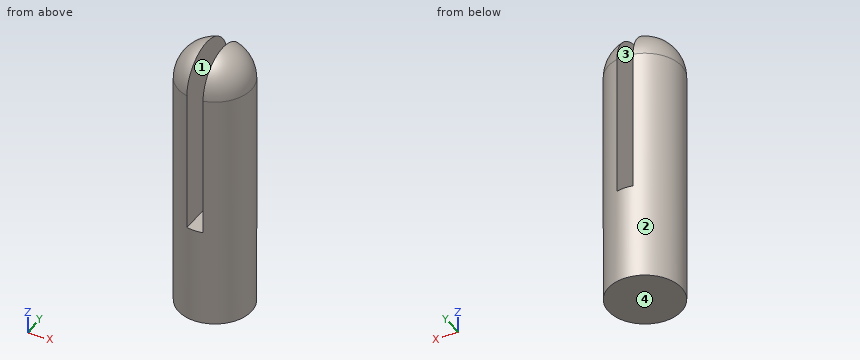
from build123d import *

# Parameters (mm, degrees)
SKETCH1_R           = 45
BOSS_EXTRUDE1_DEPTH = 340
FILLET1_R           = 45
SKETCH2_OUTSIDE_W   = 414.608
SKETCH2_OUTSIDE_H   = 164.608
SKETCH2_OUTSIDE_W_2 = 150
SKETCH2_OUTSIDE_H_2 = 90
CUT_EXTRUDE1_DEPTH  = 10


with BuildPart() as part:
    # Sketch1 → Boss-Extrude1 (new body)
    with BuildSketch(Plane.XY):
        Circle(SKETCH1_R)
    extrude(amount=BOSS_EXTRUDE1_DEPTH)

    # Fillet1
    fillet1_edges = [part.edges().sort_by_distance(p)[0] for p in [
        (-45, 0, 340),
    ]]
    fillet(fillet1_edges, radius=FILLET1_R)

    # Sketch2 outside → Cut-Extrude1 (cut, symmetric)
    with BuildSketch(Plane(origin=(0, 0, 0), x_dir=(0, 0, -1), z_dir=(1, 0, 0))):
        with Locations((-170, 0)):
            Rectangle(SKETCH2_OUTSIDE_W, SKETCH2_OUTSIDE_H)
        with Locations((-45, 0)):
            Rectangle(SKETCH2_OUTSIDE_W_2, SKETCH2_OUTSIDE_H_2, mode=Mode.SUBTRACT)
    extrude(amount=CUT_EXTRUDE1_DEPTH, both=True, mode=Mode.SUBTRACT)


solid = part.part
For this review, take the finished solid that the model builds, in its own axes (mm). Face numbers are marked on the shaded views. Coordinates: 2 decimals unless noted, no trailing zeros. Order: outer loops, then holes, each group sorted by start corner. A loop starts at its lowest first (then second) coordinate and runs counter-clockwise, first axis right, second up. Notation, with made-up numbers: (-15, 59.5) - (29, 59.5) arc R26 cw to (29, 77.5) - close; hole circle Ø9 at (54, 53.25). An arc over 180 degrees is marked (long way). Use one line per item in the form item = value.
Q1. Draft analysis for pull direction X (two halves, no side actions). For the marked faces 1, 2, 3 and 4, state which applies: +X half, -X half, draft (parallel to the pull), parting line (faces both ways), or undercut.
Checked values:
face_1 = undercut
face_2 = parting line
face_3 = undercut
face_4 = draft
Q2. Consider section A-A (y = 0). Give the boundary of the cut face in (x, z).
Checked values:
outline = (-45, 0) - (45, 0) - (45, 295) arc R45 ccw to (10, 338.87) - (10, 120) - (-10, 120) - (-10, 338.87) arc R45 ccw to (-45, 295) - close
Q3. For P1, Ø4, axis at x = -14.5, y = 21, coming from the -Z side; P2, Ø1.5, axis at x = -4, y = -25, coming from the +Z side; P3, Ø6, axis at x = 10, z = 34.5, coming from the +Y side; P4, Ø3, axis at x = -15.5, y = -29, coming from the +Z side, all flat-tipped, find the tip position at first contact; note any pin that passes through.
Checked values:
P1 = 0
P2 = 120
P3 = 44.45
P4 = 327.25
Q4. Consider section B-B (z = 209). Give the boundary of the cut face in (x, y).
Checked values:
outline = (-10, -43.87) - (-10, 43.87) arc R45 ccw to start; (10, -43.87) arc R45 ccw to (10, 43.87) - close
Q5. For probe 1 along X at (y, z) = (1, 166.5); probe 2 along X at (y, z) = (32, 149.5); probe 3 along Z at (x, y) = (1, 1), list the stretches that pass through material, from the lowest coordinate up. Write a range as from..to.
Checked values:
probe_1 = -44.99..-10, 10..44.99
probe_2 = -31.64..-10, 10..31.64
probe_3 = 0..120
Q6. Consider section C-C (x = -36). Give the boundary of the cut face in (y, z), then the cut area to 3 significant figures.
Checked values:
outline = (-27, 0) - (27, 0) - (27, 295) arc R27 ccw to (-27, 295) - close
area = 17,100 mm2
Q7. Consider section D-D (z = 25.5). Give the boundary of the cut face in (x, y).
Checked values:
outline = circle Ø90 at (0, 0)
